For this review, take the finished solid that the model builds, in its own axes (mm). A direction names the side the tool comes from. Coordinates: 2 decimals unless noted, no trailing zeros. Loops run counter-clockwise (first coordinate to the right, second up) from the corner with the lowest first, then second, coordinate; pieces in that order, holes last.
```python
from build123d import *

# Parameters (mm, degrees)
SKETCH_W        = 32
SKETCH_H        = 27
SKETCH_R        = 1.65
PAD_DEPTH       = 3
SKETCH001_R     = 5
PAD001_DEPTH    = 32
SKETCH002_R     = 1.6
POCKET_DEPTH    = 19.894216
SKETCH003_R     = 3.25
POCKET001_DEPTH = 16.894216
CHAMFER_SIZE    = 1
CHAMFER001_SIZE = 1
SKETCH004_R     = 1.25
POCKET002_DEPTH = 20.001


with BuildPart() as part:
    # Sketch → Pad (new body)
    with BuildSketch(Plane.XY):
        Rectangle(SKETCH_W, SKETCH_H)
        with Locations((-10, -10)):
            Circle(SKETCH_R, mode=Mode.SUBTRACT)
        with Locations((-10, 10)):
            Circle(SKETCH_R, mode=Mode.SUBTRACT)
        with Locations((10, 10)):
            Circle(SKETCH_R, mode=Mode.SUBTRACT)
        with Locations((10, -10)):
            Circle(SKETCH_R, mode=Mode.SUBTRACT)
    extrude(amount=PAD_DEPTH)

    # Sketch001 (on Face2 of Pad) → Pad001 (join)
    with BuildSketch(Plane.YZ.offset(16)):
        with BuildLine():
            ThreePointArc((7.5, 12.393216), (0, 19.893216), (-7.5, 12.393216))
            Line((-7.5, 12.393216), (-13.5, 0))
            Line((-13.5, 0), (13.5, 0))
            Line((7.5, 12.393216), (13.5, 0))
        make_face()
        with Locations((0, 12.393216)):
            Circle(SKETCH001_R, mode=Mode.SUBTRACT)
    extrude(amount=-PAD001_DEPTH)

    # Sketch002 (on Face4 of Pad001) → Pocket (cut, through all)
    with BuildSketch(Plane(origin=(0, 0, 0), x_dir=(1, 0, 0), z_dir=(0, 0, -1))):
        with Locations((10, 10)):
            Circle(SKETCH002_R)
        with Locations((-10, 10)):
            Circle(SKETCH002_R)
        with Locations((-10, -10)):
            Circle(SKETCH002_R)
        with Locations((10, -10)):
            Circle(SKETCH002_R)
    extrude(amount=-POCKET_DEPTH, mode=Mode.SUBTRACT)

    # Sketch003 (on Face18 of Pocket) → Pocket001 (cut, through all)
    with BuildSketch(Plane.XY.offset(3)):
        with Locations((-10, 10)):
            Circle(SKETCH003_R)
        with Locations((10, 10)):
            Circle(SKETCH003_R)
        with Locations((-10, -10)):
            Circle(SKETCH003_R)
        with Locations((10, -10)):
            Circle(SKETCH003_R)
    extrude(amount=POCKET001_DEPTH, mode=Mode.SUBTRACT)

    # Chamfer
    chamfer_edges = [part.edges().sort_by_distance(p)[0] for p in [
        (16, -5, 12.393216),
    ]]
    chamfer(chamfer_edges, length=CHAMFER_SIZE)

    # Chamfer001
    chamfer001_edges = [part.edges().sort_by_distance(p)[0] for p in [
        (-16, -5, 12.393216),
    ]]
    chamfer(chamfer001_edges, length=CHAMFER001_SIZE)

    # Sketch004 → Pocket002 (cut, through all)
    with BuildSketch(Plane.XY.offset(20)):
        Circle(SKETCH004_R)
    extrude(amount=-POCKET002_DEPTH, mode=Mode.SUBTRACT)


solid = part.part
```
Q1. Consider section A-A (x = 10). State the section outline as (y, z) points.
Q2. Consider section C-C (z = 1.25). State the section outline as (x, y) points.
Q3. The part is to be moulded in two halves that separate along Y. For faces 3 (the face through (0.111, 9.742, 7.762)), 4 (the face through (0.2, -2.4, 19.5)), 5 (the face through (10.1, -6.75, 7.84)), 6 (the face through (9.9, 6.75, 7.84)), say which applies: +Y half, -Y half, draft (parallel to the pull), parting line (faces both ways), or undercut.
Q4. Consider section B-B (y = 10). State the section outline as (x, z) points, then the cut area to 3 significant figures.
Q5. Machinability: for faces 1 (the face through (-10.1, 6.75, 7.84)), 2 (the face through (0, -13.5, 1)), which of the approach directions +Z, -Z, +X, -X, +Y, -Y give a long, thin tool a straight path to every point of the face, cutting with its end or side? Answer none if there is none.
Q6. For pin 1 Ø4 at (x, y) = (-10, 10) entering from +Z; pin 2 Ø1 at (x, z) = (-6.5, 12.5) entering from +Y; pin 3 Ø6 at (x, z) = (0, 12.5) entering from +Y, all flat-tipped, find the tip position at first contact; note any pin that passes through.
Q7. Wall thickness on probe 1 along Y at (x, z) = (10, 1.85); probe 2 along Z at (x, y) = (12.5, -9.25); probe 3 along Z at (x, y) = (-4, 0.5): over which ranges is each line inside the solid? List them lowest first.
Q8. Consider section D-D (x = 4). State the section outline as (y, z) points.
Model answer:
1. outline: (-13.5, 0) - (-11.6, 0) - (-11.6, 3) - (-13.5, 3) - close; (-8.4, 0) - (8.4, 0) - (8.4, 3) - (6.75, 3) - (6.75, 15.66) arc R7.5 ccw to (-6.75, 15.66) - (-6.75, 3) - (-8.4, 3) - close; (11.6, 0) - (13.5, 0) - (13.5, 3) - (11.6, 3) - close; hole circle Ø10 at (0, 12.39)
2. outline: (-16, -13.5) - (16, -13.5) - (16, 13.5) - (-16, 13.5) - close; hole circle Ø3.2 at (-10, -10); hole circle Ø3.2 at (-10, 10); hole circle Ø2.5 at (0, 0); hole circle Ø3.2 at (10, -10); hole circle Ø3.2 at (10, 10)
3. face 3: +Y half
3. face 4: parting line
3. face 5: undercut
3. face 6: undercut
4. outline: (-16, 0) - (-11.6, 0) - (-11.6, 3) - (-13.25, 3) - (-13.25, 7.23) - (-16, 7.23) - close; (-8.4, 0) - (8.4, 0) - (8.4, 3) - (6.75, 3) - (6.75, 7.23) - (-6.75, 7.23) - (-6.75, 3) - (-8.4, 3) - close; (11.6, 0) - (16, 0) - (16, 7.23) - (13.25, 7.23) - (13.25, 3) - (11.6, 3) - close
4. area: 157 mm2
5. face 1: +Z
5. face 2: +Z, -Z, +X, -X, -Y
6. pin 1: stops at z = 3
6. pin 2: stops at y = 7.69
6. pin 3: stops at y = 8.9
7. probe 1: y = -13.5 to -11.6, -8.4 to 8.4, 11.6 to 13.5
7. probe 2: z = 0 to 3
7. probe 3: z = 0 to 7.42, 17.37 to 19.88
8. outline: (-13.5, 0) - (13.5, 0) - (13.5, 3) - (12.05, 3) - (7.5, 12.39) arc R7.5 ccw to (-7.5, 12.39) - (-12.05, 3) - (-13.5, 3) - close; hole circle Ø10 at (0, 12.39)
